Verification items for the finished model (mm, model axes). Face numbers are marked on the shaded views. A direction names the side the tool comes from. Round coordinates to 2 decimals unless told otherwise and drop trailing zeros. Write each loop counter-clockwise with the first axis right and the second up, starting at its lowest first coordinate (ties: lowest second). Pieces come first, ordered by that corner, then holes. Notation, with made-up numbers: (88, -26) - (110, -26) arc R12 ccw to (110, -18) - close; hole circle Ø6 at (86.25, 14). An arc over 180 degrees is marked (long way). Answer as a JSON object with one key per item and string values.
```python
from build123d import *

# Parameters (mm, degrees)
F1_DEPTH  = 7.62
F3_DEPTH  = 50.8
F4_W      = 45.72
F4_H      = 38.1
F4_H_2    = 7.62
F5_DEPTH  = 7.62
F7_DEPTH  = 50.8
F8_W      = 3.81
F8_H      = 38.1
F9_DEPTH  = 25.4
F10_W     = 38.1
F10_H     = 3.81
F11_DEPTH = 38.1


with BuildPart() as f1:
    # F0 (on Top) → F1 (new body)
    with BuildSketch(Plane.XY):
        Polygon((-48.29051, -3.241779), (-55.91051, -3.241779), (-55.91051, -41.341779), (-10.19051, -41.341779), (-10.19051, -3.241779), (-17.81051, -3.241779), (-17.81051, -33.721779), (-48.29051, -33.721779), align=None)
    extrude(amount=F1_DEPTH)

    # F2 (on face) → F3 (cut)
    with BuildSketch(Plane.YZ.offset(-10.19051)):
        Polygon((-3.241779, 0), (-3.241779, 7.62), (-10.861779, 0), align=None)
    extrude(amount=-F3_DEPTH, mode=Mode.SUBTRACT)

    # F4 (on face) → F5 (join)
    with BuildSketch(Plane.XZ.offset(41.341779)):
        with Locations((-33.05051, 26.67)):
            Rectangle(F4_W, F4_H)
        with Locations((-33.05051, 3.81)):
            Rectangle(F4_W, F4_H_2)
    extrude(amount=F5_DEPTH)

    # F6 (on face) → F7 (cut)
    with BuildSketch(Plane.YZ.offset(-10.19051)):
        with BuildLine():
            Line((-48.961779, 45.72), (-48.961779, 0))
            ThreePointArc((-48.961779, 0), (-43.483086, 16.124917), (-41.341779, 33.02))
            Line((-41.341779, 33.02), (-41.341779, 45.72))
            Line((-41.341779, 45.72), (-48.961779, 45.72))
        make_face()
    extrude(amount=-F7_DEPTH, mode=Mode.SUBTRACT)

    # F8 (on face) → F9 (join)
    with BuildSketch(Plane.XY.offset(7.62)):
        Polygon((-10.19051, -3.241779), (-10.19051, -41.341779), (-6.38051, -22.291779), align=None)
        with Locations((-12.09551, -22.291779)):
            Rectangle(F8_W, F8_H)
        with Locations((-54.00551, -22.291779)):
            Rectangle(F8_W, F8_H)
        Polygon((-59.72051, -22.291779), (-55.91051, -41.341779), (-55.91051, -3.241779), align=None)
    extrude(amount=F9_DEPTH)

    # F10 (on face) → F11 (join)
    with BuildSketch(Plane.YZ.offset(-52.10051)):
        with Locations((-22.291779, 24.765)):
            Rectangle(F10_W, F10_H)
    extrude(amount=F11_DEPTH)


solid = f1.part
```
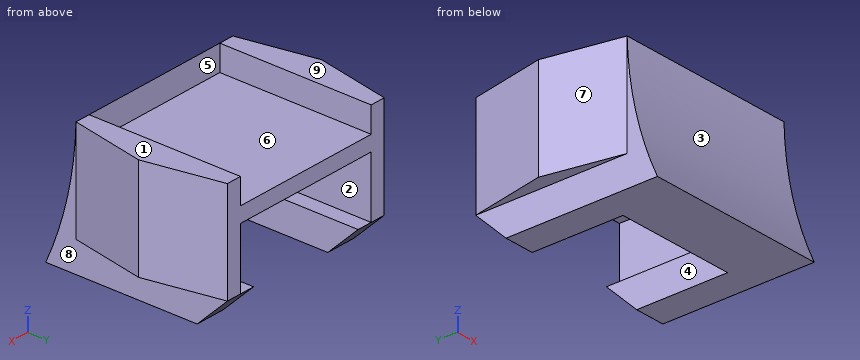
Q1. Section check B-B, the plane y = -12.5. Record the cut outline in (x, z).
Geometry check:
{"outline": "(-57.76, 7.62) - (-55.91, 7.62) - (-55.91, 0) - (-48.29, 0) - (-48.29, 7.62) - (-52.1, 7.62) - (-52.1, 22.86) - (-14, 22.86) - (-14, 7.62) - (-17.81, 7.62) - (-17.81, 0) - (-10.19, 0) - (-10.19, 7.62) - (-8.34, 7.62) - (-8.34, 33.02) - (-14, 33.02) - (-14, 26.67) - (-52.1, 26.67) - (-52.1, 33.02) - (-57.76, 33.02) - close"}
Q2. Release check for a two-part mould opening along X. For the marked faces 6, 7, 8 and 9 record: released by +X, released by -X, zero draft, split by the parting line, or undercut.
Geometry check:
{"face 6": "undercut", "face 7": "released by -X", "face 8": "released by +X", "face 9": "zero draft"}
Q3. Material ranges on line 1 along Z through (x, y) = (-15, -31); line 2 along X through (y, z) = (-16.5, 3); line 3 along X through (y, z) = (-37.5, 27), recorded low to high. Write a range as [from, to].
Geometry check:
{"line 1": "z = [0, 7.62], [22.86, 26.67]", "line 2": "x = [-55.91, -48.29], [-17.81, -10.19]", "line 3": "x = [-56.68, -52.1], [-14, -9.42]"}
Q4. Gauge pin test, flat ends, axial feed: P1, Ø8, axis at y = -34, z = 21, coming from the +X side; P2, Ø7.5, axis at y = -18.5, z = 15, coming from the -X side; P3, Ø3, axis at x = -27.5, y = -34.5, coming from the +Z side. Record the tip position at first contact, or that the pin passes through.
Geometry check:
{"P1": "stops at x = -7.92", "P2": "stops at x = -59.71", "P3": "stops at z = 26.67"}
Q5. Section check C-C, the plane z = 14.5. Record the cut outline in (x, y) (1 decimal), then the cut area to 3 significant figures.
Geometry check:
{"outline": "(-59.7, -22.3) - (-55.9, -41.3) - (-55.9, -43.9) - (-10.2, -43.9) - (-10.2, -41.3) - (-6.4, -22.3) - (-10.2, -3.2) - (-14, -3.2) - (-14, -41.3) - (-52.1, -41.3) - (-52.1, -3.2) - (-55.9, -3.2) - close", "area": "551 mm2"}
Q6. Section check D-D, the plane y = -40.5. Record the cut outline in (x, z), then the cut area to 3 significant figures.
Geometry check:
{"outline": "(-56.08, 7.62) - (-55.91, 7.62) - (-55.91, 0) - (-10.19, 0) - (-10.19, 7.62) - (-10.02, 7.62) - (-10.02, 33.02) - (-14, 33.02) - (-14, 26.67) - (-52.1, 26.67) - (-52.1, 33.02) - (-56.08, 33.02) - close; hole (-52.1, 7.62) - (-14, 7.62) - (-14, 22.86) - (-52.1, 22.86) - close", "area": "696 mm2"}
Q7. Set-up check for the marked faces 1, 2, 3, 4 and 5: record each of +Z, -Z, +X, -X, +Y, -Y from which the full face is reachable in a straight line by a thin tool's end or side.
Geometry check:
{"face 1": "+Z, +X, -X, +Y, -Y", "face 2": "+Y", "face 3": "+Z, +X, -X, -Y", "face 4": "-Z, +Y", "face 5": "+Z, +Y"}
Q8. Section check A-A, the plane x = -45.5. Record the cut outline in (y, z), then the cut area to 3 significant figures.
Geometry check:
{"outline": "(-48.96, 0) - (-33.72, 0) - (-33.72, 7.62) - (-41.34, 7.62) - (-41.34, 22.86) - (-3.24, 22.86) - (-3.24, 26.67) - (-41.34, 26.67) - (-41.34, 33.02) arc R84.68 cw to start", "area": "290 mm2"}
